from build123d import *

# Parameters (mm, degrees)
SKETCH_1_W          = 18.38477631
SKETCH_1_H          = 18.38477631
EXTRUDE_2_DEPTH     = 14
SKETCH_5_W          = 26
SKETCH_5_H          = 34
EXTRUDE_4_DEPTH     = 2
SKETCH_6_R          = 1.5
CUT_EXTRUDE_1_DEPTH = 2


with BuildPart() as part:
    # 草图1 → 凸台-拉伸2 (new body)
    with BuildSketch(Plane(origin=(0, 0, 0), x_dir=(0, 0, -1), z_dir=(1, 0, 0))):
        with Locations((0, 1.25)):
            Rectangle(SKETCH_1_W, SKETCH_1_H)
    extrude(amount=EXTRUDE_2_DEPTH)

    # 草图5 → 凸台-拉伸4 (add)
    with BuildSketch(Plane.ZY):
        Rectangle(SKETCH_5_W, SKETCH_5_H)
    extrude(amount=EXTRUDE_4_DEPTH)

    # 草图6 → 切除-拉伸1 (cut)
    with BuildSketch(Plane(origin=(0, 0, 0), x_dir=(0, 0, -1), z_dir=(1, 0, 0))):
        with Locations((-10, 14)):
            Circle(SKETCH_6_R)
        with Locations((10, 14)):
            Circle(SKETCH_6_R)
        with Locations((-10, -14)):
            Circle(SKETCH_6_R)
        with Locations((10, -14)):
            Circle(SKETCH_6_R)
    extrude(amount=-CUT_EXTRUDE_1_DEPTH, mode=Mode.SUBTRACT)


solid = part.part
CAD build for the part. Positions are in the model's coordinates, mm. A direction names the side the tool comes from. Give positions to 0.01 mm unless a question says otherwise; leave off trailing zeros. Loops run counter-clockwise (first coordinate to the right, second up) from the corner with the lowest first, then second, coordinate; pieces in that order, holes last. Notation, with made-up numbers: M 70,-8 L 78,-8 A19 ccw 78,10 Z; hole C 29.25,47.5 d8. An arc over 180 degrees is marked long. Answer in a Markdown table with one row per item. Add a question column.
Item 1: Band-saw the part on D-D on z = 3. Give the cut face in (x, y).
Item 2: Probe probe 1 along Y at (x, z) = (-1.25, -10); probe 2 along Y at (x, z) = (2.25, 8.25); probe 3 along X at (y, z) = (14, -5.75). List the from-to ranges inside material, lowest first.
Item 3: Band-saw the part on C-C on y = -1.5. Give the cut face in (x, z).
Item 4: Band-saw the part on B-B on y = -14. Give the cut face in (x, z), then the cut area to 3 significant figures.
Item 5: Tool access for faces 4 (the face through (-0.99, -13.93, 11.5)), 5 (the face through (7, 10.442, 0)), 6 (the face through (7, 1, -9.192)), 7 (the face through (7, 1, 9.192)): list every direction of +Z, -Z, +X, -X, +Y, -Y with a clear straight run to the whole face (end or side of a thin tool).
Item 6: Drop flat-ended pins along their axis: P1, Ø2.5, axis at y = -14, z = 10, coming from the +X side; P2, Ø3, axis at x = 11, y = 7.5, coming from the +Z side; P3, Ø6, axis at x = 5, z = 1.5, coming from the -Y side; P4, Ø4, axis at x = 4, y = 1.5, coming from the -Z side. Give the stop position or say it passes through.
Item 7: Band-saw the part on A-A on z = -10. Give the cut face in (x, y).
Item 8: Mould opens along Y. For faces 1 (the face through (14, 1, 0)), 2 (the face through (7, -7.942, 0)), 3 (the face through (-0.99, -13.93, -8.5)) say: +Y half, -Y half, draft (parallel to the pull), parting line (faces both ways), or undercut.
Reply:
| question | item | result |
|---|---|---|
| 1 | outline | M -2,-17 L 0,-17 L 0,-7.94 L 14,-7.94 L 14,10.44 L 0,10.44 L 0,17 L -2,17 Z |
| 2 | probe 1 | y = -17 to -15.5, -12.5 to 12.5, 15.5 to 17 |
| 2 | probe 2 | y = -7.94 to 10.44 |
| 2 | probe 3 | x = -2 to 0 |
| 3 | outline | M -2,-13 L 0,-13 L 0,-9.19 L 14,-9.19 L 14,9.19 L 0,9.19 L 0,13 L -2,13 Z |
| 4 | outline | M -2,-13 L 0,-13 L 0,-11.5 L -2,-11.5 Z; M -2,-8.5 L 0,-8.5 L 0,8.5 L -2,8.5 Z; M -2,11.5 L 0,11.5 L 0,13 L -2,13 Z |
| 4 | area | 40.0 mm^2 |
| 5 | face 4 | +X, -X |
| 5 | face 5 | +Z, -Z, +X, +Y |
| 5 | face 6 | -Z, +X, +Y, -Y |
| 5 | face 7 | +Z, +X, +Y, -Y |
| 6 | P1 | passes through |
| 6 | P2 | stops at z = 9.19 |
| 6 | P3 | stops at y = -7.94 |
| 6 | P4 | stops at z = -9.19 |
| 7 | outline | M -2,-17 L 0,-17 L 0,-15.5 L -2,-15.5 Z; M -2,-12.5 L 0,-12.5 L 0,12.5 L -2,12.5 Z; M -2,15.5 L 0,15.5 L 0,17 L -2,17 Z |
| 8 | face 1 | draft |
| 8 | face 2 | -Y half |
| 8 | face 3 | undercut |
